For this review, take the finished solid that the model builds, in its own axes (mm). A direction names the side the tool comes from. Coordinates: 2 decimals unless noted, no trailing zeros. Loops run counter-clockwise (first coordinate to the right, second up) from the corner with the lowest first, then second, coordinate; pieces in that order, holes last. Notation, with made-up numbers: (67.25, 5.5) -> (124.25, 5.5) arc R28 cw to (124.25, 42.5) -> close; hole circle Ø1 at (88.25, -39). An arc over 180 degrees is marked (long way). One line per item, written item: value.
from build123d import *

# Parameters (mm, degrees)
BOSS_EXTRUDE1_DEPTH = 90
SHELL1_T            = -1
SKETCH2_W           = 5
SKETCH2_H           = 2.5
CUT_EXTRUDE2_DEPTH  = 3


with BuildPart() as part:
    # Sketch1 → Boss-Extrude1 (new body)
    with BuildSketch(Plane(origin=(0, 0, 0), x_dir=(0, 0, -1), z_dir=(1, 0, 0))):
        with BuildLine():
            Line((0, 0), (0.468395453, 1.431403189))
            ThreePointArc((0.468395453, 1.431403189), (2.268780711, 3.308334479), (4.858963514, 3.073363867))
            Line((4.858963514, 3.073363867), (10, 0))
            Line((10, 0), (0, 0))
        make_face()
    extrude(amount=BOSS_EXTRUDE1_DEPTH)

    # Shell1
    shell1_openings = [part.faces().sort_by_distance(p)[0] for p in [
        (45, 0, -5),
    ]]
    offset(amount=SHELL1_T, openings=shell1_openings, kind=Kind.INTERSECTION)

    # Sketch2 → Cut-Extrude2 (cut)
    with BuildSketch(Plane(origin=(0, 0, 0), x_dir=(1, 0, 0), z_dir=(0, 0.311000813, 0.950409645))):
        with Locations((4.5, 2.756090765)):
            Rectangle(SKETCH2_W, SKETCH2_H)
        with Locations((14.5, 2.756090765)):
            Rectangle(SKETCH2_W, SKETCH2_H)
        with Locations((24.5, 2.756090765)):
            Rectangle(SKETCH2_W, SKETCH2_H)
        with Locations((34.5, 2.756090765)):
            Rectangle(SKETCH2_W, SKETCH2_H)
        with Locations((44.5, 2.756090765)):
            Rectangle(SKETCH2_W, SKETCH2_H)
        with Locations((54.5, 2.756090765)):
            Rectangle(SKETCH2_W, SKETCH2_H)
        with Locations((64.5, 2.756090765)):
            Rectangle(SKETCH2_W, SKETCH2_H)
        with Locations((74.5, 2.756090765)):
            Rectangle(SKETCH2_W, SKETCH2_H)
        with Locations((84.5, 2.756090765)):
            Rectangle(SKETCH2_W, SKETCH2_H)
    extrude(amount=-CUT_EXTRUDE2_DEPTH, mode=Mode.SUBTRACT)


solid = part.part
1. Take a section at B-B, the plane z = -6.5. Give the boundary of the cut face in (x, y), and give its area (3 significant figures).
Return value:
outline: (0, 0) -> (1, 0) -> (1, 0.93) -> (89, 0.93) -> (89, 0) -> (90, 0) -> (90, 2.09) -> (0, 2.09) -> close
area: 107 mm2
2. The part is to be moulded in two halves that separate along X. For faces 3 (the flat face through (52, 3, -2)), 4 (the flat face through (45, 0, -9)), say which applies: pulls with the +X half, pulls with the -X half, needs draft (parallel to the pull), parting line crosses it, or undercut.
Return value:
face 3: undercut
face 4: needs draft
3. To check wall thickness, follow probe 1 along X at (y, z) = (0.3, -2.5); probe 2 along Y at (x, z) = (85.5, -3.5); probe 3 along Z at (x, y) = (8.5, 0.9). State the ranges of each line that lie inside material, in increasing order. Write a range as from..to.
Return value:
probe 1: x = 0..1, 89..90
probe 2: y = 3.07..3.49
probe 3: z = -8.49..-6.55, -1.35..-0.29
4. Take a section at A-A, the plane x = 54. Give the boundary of the cut face in (y, z).
Return value:
outline: (0, -10) -> (3.07, -4.86) arc R3 ccw to (3.39, -2.52) -> (2.87, -4.1) -> (2.4, -3.94) arc R2 cw to (2.22, -4.35) -> (0, -8.05) -> close; (0, -1.05) -> (1.12, -1.42) -> (1.43, -0.47) -> (0, 0) -> close
5. Insertion check: pin 1 Ø3 at (x, z) = (72, -5) entering from +Y. The pin has a flat end and moves straight along its axis. Give the tip position at first contact, or say it passes through.
Return value:
pin 1: stops at y = 3.49
6. For faces 1 (the flat face through (44.37, 1.56, -7.39)), 2 (the flat face through (89, 1, -4)), list the 3-axis set-ups (+Z, -Z, +X, -X, +Y, -Y) from which the entire face can be reached by the end or side of a thin tool; tool diameter is ignored.
Return value:
face 1: -Z, +X, -X, +Y
face 2: -Y
